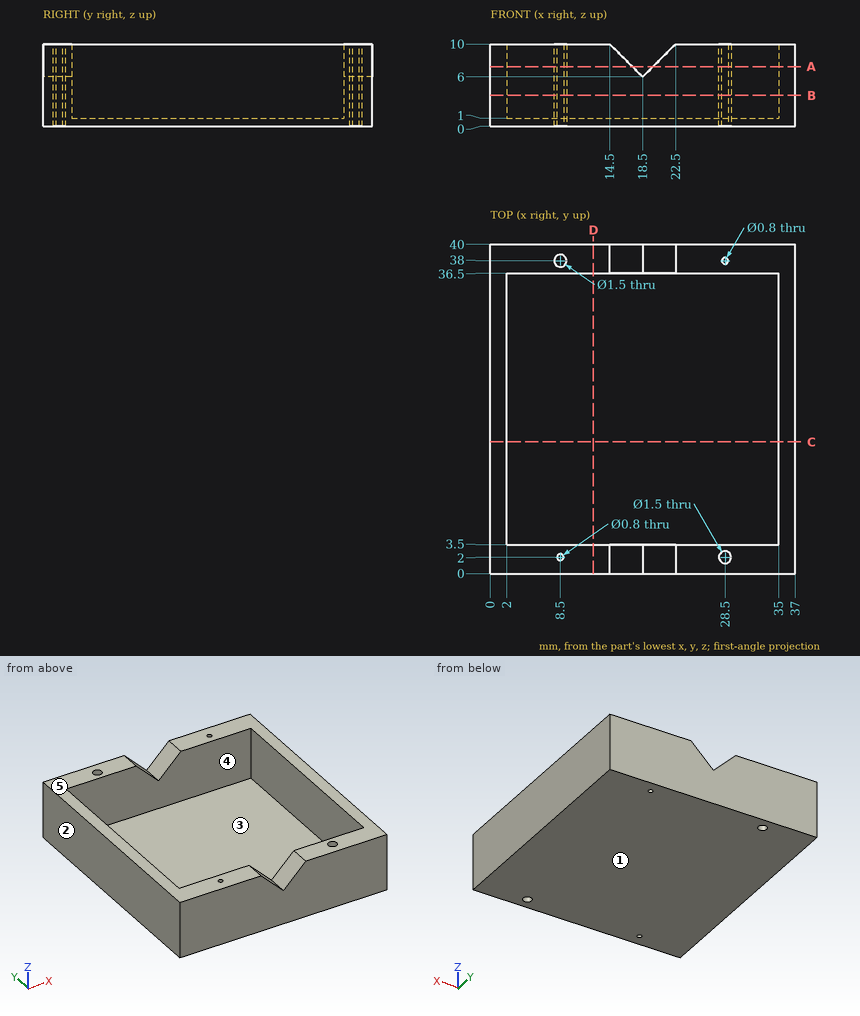
For this review, use the dimensioned drawing (mm, ordinates from the lowest corner) and the shaded views. A direction names the side the tool comes from. Round coordinates to 2 decimals unless told otherwise and drop trailing zeros. Write each loop counter-clockwise with the first axis right and the second up, starting at its lowest first coordinate (ties: lowest second). Pieces come first, ordered by that corner, then holes. Notation, with made-up numbers: (-3.75, -21) -> (20.25, -21) arc R5 cw to (20.25, -12) -> close; hole circle Ø4 at (-33.5, -34.75). An arc over 180 degrees is marked (long way). Use one line per item in the form item = value.
Q1. Consider section B-B (z = 3.75). State the section outline as (x, y) points.
Resolved:
outline = (0, 0) -> (37, 0) -> (37, 40) -> (0, 40) -> close; hole (2, 3.5) -> (35, 3.5) -> (35, 36.5) -> (2, 36.5) -> close; hole circle Ø1.5 at (8.5, 38); hole circle Ø0.8 at (8.5, 2); hole circle Ø1.5 at (28.5, 2); hole circle Ø0.8 at (28.5, 38)
Q2. Consider section A-A (z = 7.25). State the section outline as (x, y) points.
Resolved:
outline = (0, 0) -> (17.25, 0) -> (17.25, 3.5) -> (2, 3.5) -> (2, 36.5) -> (17.25, 36.5) -> (17.25, 40) -> (0, 40) -> close; (19.75, 0) -> (37, 0) -> (37, 40) -> (19.75, 40) -> (19.75, 36.5) -> (35, 36.5) -> (35, 3.5) -> (19.75, 3.5) -> close; hole circle Ø1.5 at (8.5, 38); hole circle Ø0.8 at (8.5, 2); hole circle Ø1.5 at (28.5, 2); hole circle Ø0.8 at (28.5, 38)
Q3. To check wall thickness, follow probe 1 along Y at (x, z) = (28.5, 7); probe 2 along X at (y, z) = (38, 5.5); probe 3 along Y at (x, z) = (8.5, 7). State the ranges of each line that lie inside material, in increasing order. Write a range as from..to.
Resolved:
probe_1 = 0..1.25, 2.75..3.5, 36.5..37.6, 38.4..40
probe_2 = 0..7.75, 9.25..28.1, 28.9..37
probe_3 = 0..1.6, 2.4..3.5, 36.5..37.25, 38.75..40
Q4. The part is to be moulded in two halves that separate along X. For the marked faces 1, 2 and 3, say which applies: released by +X, released by -X, zero draft, split by the parting line, or undercut.
Resolved:
face_1 = zero draft
face_2 = released by -X
face_3 = undercut
Q5. Machinability: for the marked faces 4 and 5, which of the approach directions +Z, -Z, +X, -X, +Y, -Y give a long, thin tool a straight path to every point of the face, cutting with its end or side? Answer none if there is none.
Resolved:
face_4 = +Z
face_5 = +Z, +X, -X, +Y, -Y
Q6. Clearance check with flat-ended pins moving along their axes: pin 1 Ø1.2 at (x, y) = (8.5, 38) entering from +Z; pin 2 Ø2.5 at (x, y) = (28.5, 2) entering from +Z. State where each tip first meets the part, or that it passes through.
Resolved:
pin_1 = through
pin_2 = 10
Q7. Consider section C-C (y = 16). State the section outline as (x, z) points.
Resolved:
outline = (0, 0) -> (37, 0) -> (37, 10) -> (35, 10) -> (35, 1) -> (2, 1) -> (2, 10) -> (0, 10) -> close
Q8. Consider section D-D (x = 12.5). State the section outline as (y, z) points, then the cut area to 3 significant figures.
Resolved:
outline = (0, 0) -> (40, 0) -> (40, 10) -> (36.5, 10) -> (36.5, 1) -> (3.5, 1) -> (3.5, 10) -> (0, 10) -> close
area = 103 mm²
